Autodesk Inventor part; units mm, degrees
ref_plane "YZ Plane" through (0, 0, 0) normal (1, 0, 0) x (0, 1, 0)
ref_plane "XZ Plane" through (0, 0, 0) normal (0, 1, 0) x (-1, 0, 0)
ref_plane "XY Plane" through (0, 0, 0) normal (0, 0, 1) x (1, 0, 0)
sketch "スケッチ1" plane through (0, 0, 0) normal (1, 0, 0) x (0, 1, 0)
  line L0 (-15, -16) -> (15, -16)
  line L1 (15, -16) -> (15, 16)
  line L2 (15, 16) -> (-15, 16)
  line L3 (-15, 16) -> (-15, -16)
  line L4 (-15, -16) -> (15, 16) construction
  line L5 (15, -16) -> (-15, 16) construction
  point P0 (0, 0)
  dimension "d0" = 32
  dimension "d1" = 30
extrude "押し出し1" add sketch "スケッチ1" along normal blind 14
sketch "スケッチ2" plane through (0, -15, 16) normal (0, 0, 1) x (1, 0, 0)
  line L0 (0, 30) -> (0, 0)
  line L1 (0, 0) -> (14, 0)
  line L2 (14, 30) -> (14, 0)
  line L3 (0, 30) -> (14, 30)
  circle A0 centre (6, 15) radius 3
  point P0 (0, 15)
  dimension "d4" = 6
  dimension "d17" = 6
extrude "押し出し2" cut sketch "スケッチ2" against normal through all contours A0
sketch "スケッチ3" plane through (14, 0, 0) normal (1, 0, 0) x (0, 0, -1)
  line L0 (-10, 10) -> (10, 10)
  line L1 (10, 10) -> (10, -10)
  line L2 (10, -10) -> (-10, -10)
  line L3 (-10, -10) -> (-10, 10)
  line L4 (-10, 10) -> (10, -10) construction
  line L5 (10, 10) -> (-10, -10) construction
  line L6 (-16, 15) -> (-16, -15)
  point P0 (0, 0)
  point P1 (0, 0)
  dimension "d7" = 20
  dimension "d8" = 20
  dimension "d9" = 6
hole "穴1" at (14, 10, -10) at (14, 10, 10) at (14, -10, 10) at (14, -10, -10) direction (-1, 0, 0) diameter 2.459 depth 8.8
properties part number "Linear_Unit_B"
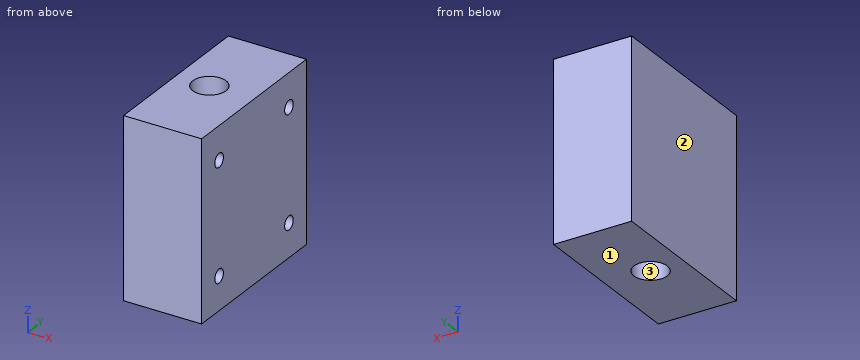
Input: part model. Units: mm. Frame: model coordinates. Face numbers are marked on the shaded views. Coordinates: 2 decimals unless noted, no trailing zeros. Write each loop counter-clockwise with the first axis right and the second up, starting at its lowest first coordinate (ties: lowest second). Pieces come first, ordered by that corner, then holes. Notation, with made-up numbers: M 51.5,37.25 L 85.5,37.25 A35 cw 85.5,75.25 Z; hole C -33.5,84 d7. An arc over 180 degrees is marked long. Answer as a JSON object with one key per item and string values. Group by question number.
(1) Section A-A on x = 6. Output: boundary loops of the cut face in (y, z), plus the area to 3 significant figures.
(2) Contact query for a flat-ended pin moving along its axis: P1, Ø2, axis at y = -10, z = 10, coming from the +X side. Output: stop coordinate, or through.
(3) Section B-B on y = 0. Output: boundary loops of the cut face in (x, z).
(4) Section C-C on z = 10. Output: boundary loops of the cut face in (x, y), plus the area to 3 significant figures.
(5) Mould query, pull axis X, two halves, no side actions, for the marked faces 1, 2 and 3. Classes: pulls with the +X half, pulls with the -X half, needs draft (parallel to the pull), parting line crosses it, or undercut.
(6) Section D-D on x = 12. Output: boundary loops of the cut face in (y, z).
(7) Ray query, line 1 along Z through (x, y) = (11.5, 10); line 2 along Y through (x, z) = (12, -10); line 3 along Y through (x, z) = (6, 3.5). Return the intervals inside material, ascending. Write a range as [from, to].
Result set:
{
 "1": {"outline": "M -15,-16 L -3,-16 L -3,16 L -15,16 Z; M 3,-16 L 15,-16 L 15,16 L 3,16 Z; hole C -10,-10 d2.46; hole C -10,10 d2.46; hole C 10,-10 d2.46; hole C 10,10 d2.46", "area": "749 mm2"},
 "2": {"P1": "stops at x = 5.2"},
 "3": {"outline": "M 0,-16 L 3,-16 L 3,16 L 0,16 Z; M 9,-16 L 14,-16 L 14,16 L 9,16 Z"},
 "4": {"outline": "M 0,-15 L 14,-15 L 14,-11.23 L 5.2,-11.23 L 5.2,-8.77 L 14,-8.77 L 14,8.77 L 5.2,8.77 L 5.2,11.23 L 14,11.23 L 14,15 L 0,15 Z; hole C 6,0 d6", "area": "348 mm2"},
 "5": {"face 1": "needs draft", "face 2": "pulls with the -X half", "face 3": "undercut"},
 "6": {"outline": "M -15,-16 L 15,-16 L 15,16 L -15,16 Z; hole C -10,-10 d2.46; hole C -10,10 d2.46; hole C 10,-10 d2.46; hole C 10,10 d2.46"},
 "7": {"line 1": "z = [-16, -11.23], [-8.77, 8.77], [11.23, 16]", "line 2": "y = [-15, -11.23], [-8.77, 8.77], [11.23, 15]", "line 3": "y = [-15, -3], [3, 15]"}
}
